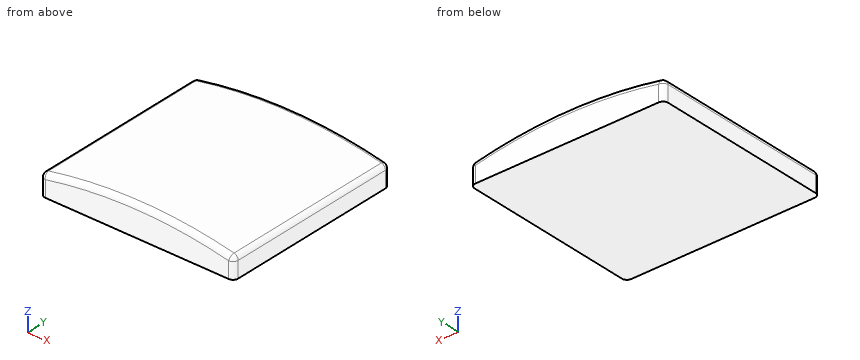
from build123d import *

# Parameters (mm, degrees)
F1_DEPTH = 228.6
F0_W     = 482.6
F0_H     = 50.8
F2_DEPTH = 228.6
F3_R     = 12.7


with BuildPart() as f1:
    # F0 (on Front) → F1 (new body, symmetric)
    with BuildSketch(Plane.XZ):
        with BuildLine():
            Line((-241.3, 25.4), (241.3, 25.4))
            ThreePointArc((241.3, 25.4), (0, 50.8), (-241.3, 25.4))
        make_face()
    extrude(amount=F1_DEPTH, both=True)

    # F0 (on Front) → F2 (join, symmetric)
    with BuildSketch(Plane.XZ):
        Rectangle(F0_W, F0_H)
        with BuildLine():
            Line((-241.3, 25.4), (241.3, 25.4))
            ThreePointArc((241.3, 25.4), (0, 50.8), (-241.3, 25.4))
        make_face()
    extrude(amount=F2_DEPTH, both=True)

    # F3
    f3_edges = [f1.edges().sort_by_distance(p)[0] for p in [
        (-241.3, 228.6, 0),
        (-241.3, -228.6, 0),
        (241.3, 228.6, 0),
        (241.3, -228.6, 0),
        (241.3, 0, 25.4),
        (0, -228.6, 50.8),
        (0, 228.6, 50.8),
        (-241.3, 0, 25.4),
    ]]
    fillet(f3_edges, radius=F3_R)


solid = f1.part
CAD build for the part. Positions are in the model's coordinates, mm. Round coordinates to 2 decimals unless told otherwise and drop trailing zeros. Order: outer loops, then holes, each group sorted by start corner. A loop starts at its lowest first (then second) coordinate and runs counter-clockwise, first axis right, second up. Notation, with made-up numbers: (-28.75, 14) - (23.25, 14) arc R21 ccw to (23.25, 34) - close; hole circle Ø10 at (75, 78). An arc over 180 degrees is marked (long way). Return JSON: item names as keys, results as strings.
(1) Pin check, flat tips, straight feed: pin 1 Ø10 at (y, z) = (-103, 23.5) entering from +X; pin 2 Ø10 at (y, z) = (-82, 22.5) entering from -X. Stop position of each tip, or through.
Answer key:
{"pin 1": "stops at x = 240.83", "pin 2": "stops at x = -241.07"}
(2) Cut at A-A (y = -100). Give the cut face in (x, z) (3 decimals).
Answer key:
{"outline": "(-241.3, -25.4) - (241.3, -25.4) - (241.3, 15.072) arc R12.7 ccw to (231.133, 27.517) arc R1158.875 ccw to (-231.133, 27.517) arc R12.7 ccw to (-241.3, 15.072) - close"}
(3) Wall check: probe 1 along Y at (x, z) = (-3.5, 40.5); probe 2 along Z at (x, y) = (214, -146); probe 3 along Y at (x, z) = (143.5, 30). Give the ranges that are in metal, low to high. Write a range as from..to.
Answer key:
{"probe 1": "y = -228.37..228.37", "probe 2": "z = -25.4..30.87", "probe 3": "y = -228.57..228.57"}
